Read the model definition and answer for the solid it produces. Units are mm, in the model's axes. A direction names the side the tool comes from. Give positions to 0.01 mm unless a question says otherwise; leave off trailing zeros. Order: outer loops, then holes, each group sorted by start corner. A loop starts at its lowest first (then second) coordinate and runs counter-clockwise, first axis right, second up.
```python
from build123d import *

# Parameters (mm, degrees)
F1_DEPTH = 73


with BuildPart() as f1:
    # F0 (on Top) → F1 (new body)
    with BuildSketch(Plane.XY):
        with BuildLine():
            Line((-72.7140201691, 8.0667017028), (-131.6497474909, 8.0667017028))
            Line((-131.6497474909, 8.0667017028), (-131.6497474909, -19.9154652655))
            Line((-131.6497474909, -19.9154652655), (-65.753698349, -19.9154652655))
            Line((-65.753698349, -19.9154652655), (-65.753698349, -8.1091851911))
            ThreePointArc((-65.753698349, -8.1091851911), (-70.0204713157, -0.3597130192), (-72.7140201691, 8.0667017028))
        make_face()
        with BuildLine():
            ThreePointArc((12.0841842232, 39.5514563587), (-43.95195039, 60.5378347362), (-72.7140201691, 8.0667017028))
            Line((-72.7140201691, 8.0667017028), (-65.753698349, 8.0667017028))
            Line((-65.753698349, 8.0667017028), (-65.753698349, -8.1091851911))
            ThreePointArc((-65.753698349, -8.1091851911), (-50.4399597526, -22.1300637719), (-30.5028123826, -27.9271130837))
            ThreePointArc((-30.5028123826, -27.9271130837), (-34.9735728703, 22.0724808102), (12.0841842232, 39.5514563587))
        make_face()
        with BuildLine():
            Line((-65.753698349, 8.0667017028), (-72.7140201691, 8.0667017028))
            ThreePointArc((-72.7140201691, 8.0667017028), (-70.0204713157, -0.3597130192), (-65.753698349, -8.1091851911))
            Line((-65.753698349, -8.1091851911), (-65.753698349, 8.0667017028))
        make_face()
        with BuildLine():
            ThreePointArc((41.3563200543, 0), (33.2423118838, 24.6027215782), (12.0841842232, 39.5514563587))
            ThreePointArc((12.0841842232, 39.5514563587), (16.234552473, 28.9747517123), (17.6471201799, 17.7010260522))
            ThreePointArc((17.6471201799, 17.7010260522), (3.3833749523, -15.4665148831), (-30.5028123826, -27.9271130837))
            ThreePointArc((-30.5028123826, -27.9271130837), (14.9810069252, -38.5475633464), (41.3563200543, 0))
        make_face()
        with BuildLine():
            ThreePointArc((17.6471201799, 17.7010260522), (16.234552473, 28.9747517123), (12.0841842232, 39.5514563587))
            ThreePointArc((12.0841842232, 39.5514563587), (-34.9735728703, 22.0724808102), (-30.5028123826, -27.9271130837))
            ThreePointArc((-30.5028123826, -27.9271130837), (3.3833749523, -15.4665148831), (17.6471201799, 17.7010260522))
        make_face()
    extrude(amount=F1_DEPTH)


solid = f1.part
```
1) A tool of negligible diameter and unlimited length cuts with its end or side. For faces 1 (the face through (-27, 12, 0)), 2 (the face through (-99, -19.915, 36)), from which of +Z, -Z, +X, -X, +Y, -Y can it reach the whole face along a straight path? Write none if from no direction.
Final values:
face 1: -Z, +X, -X, +Y, -Y
face 2: +Z, -Z, -X, -Y
2) Consider L1, parallel to Y at x = -79, z = 60; L2, parallel to Y at x = -28, z = 20.5; L3, parallel to X at y = 15, z = 41. Determine where each line is inside the solid, lowest interval first.
Final values:
L1: y = -19.92 to 8.07
L2: y = -30.44 to 63.4
L3: x = -73.66 to 38.54
3) The part is cut by section A-A on z = 57. Determine the outline of the cut face in (x, y).
Final values:
outline: (-131.65, -19.92) - (-65.75, -19.92) - (-65.75, -8.11) arc R45.69 ccw to (-30.5, -27.93) arc R41.36 ccw (long way) to (12.08, 39.55) arc R45.69 ccw to (-72.71, 8.07) - (-131.65, 8.07) - close
4) The part is cut by section C-C on y = 37. Determine the outline of the cut face in (x, z), and give its area (3 significant figures).
Final values:
outline: (-69.47, 0) - (18.48, 0) - (18.48, 73) - (-69.47, 73) - close
area: 6,420 mm2
5) Given pin 1 (4 mm diameter, centred on y = -15, z = 57, fed in from +X); pin 2 (1.5 mm diameter, centred on x = -5.5, z = 11.5, fed in from -Y); pin 3 (8 mm diameter, centred on y = 47, z = 38.5, fed in from -X), each flat-ended and moving along its own axis, determine where each tip first touches the part or whether it passes through.
Final values:
pin 1: stops at x = 39.26
pin 2: stops at y = -41.08
pin 3: stops at x = -66.1
6) For a pull along X with two mould halves and no side action, classify faces 3 (the face through (-27, 12, 73)), 4 (the face through (-131.65, -6, 36)), 5 (the face through (-50.695, -21.986, 35.989)) as released by +X, released by -X, zero draft, split by the parting line, or undercut.
Final values:
face 3: zero draft
face 4: released by -X
face 5: undercut
7) The part is cut by section B-B on x = -97. Determine the outline of the cut face in (y, z).
Final values:
outline: (-19.92, 0) - (8.07, 0) - (8.07, 73) - (-19.92, 73) - close
